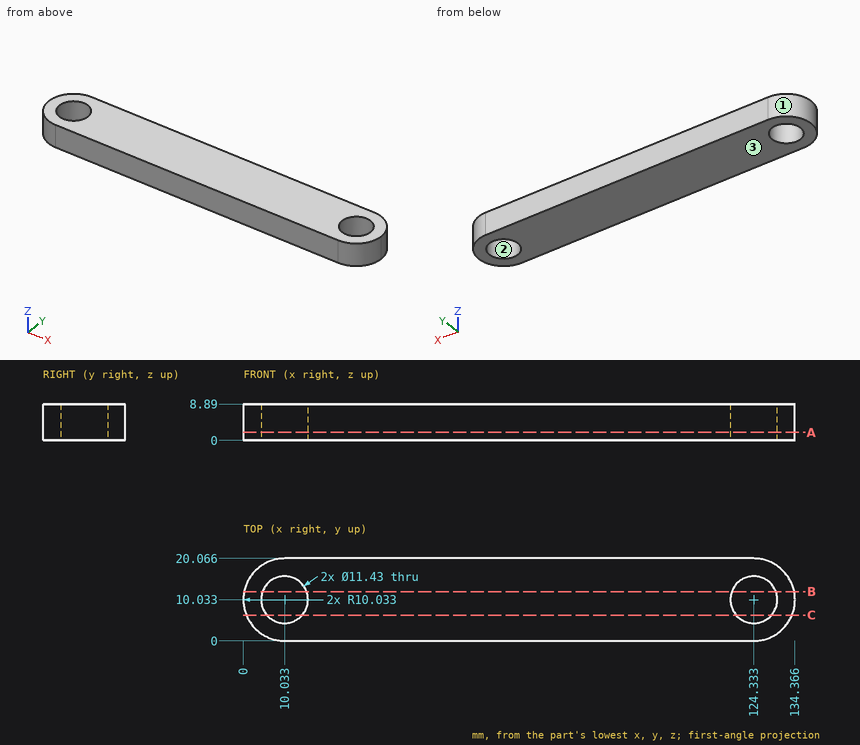
Input: dimensioned drawing with shaded views. Units: mm. Origin: part minimum x, y, z. Give positions to 0.01 mm unless a question says otherwise; leave off trailing zeros. Write each loop counter-clockwise with the first axis right and the second up, starting at its lowest first coordinate (ties: lowest second). Pieces come first, ordered by that corner, then holes. Notation, with made-up numbers: M -32.75,23.5 L 9.25,23.5 A24 cw 9.25,51.5 Z; hole C 60,-36 d3. An arc over 180 degrees is marked long. Write item = value, one per line. Start each with the question number.
1) Material intervals for line 1 along X through (y, z) = (5.5, 5.25); line 2 along X through (y, z) = (7, 7); line 3 along Y through (x, z) = (13, 2.5), sorted ascending. Write a range as [from, to].
2) Draft query along X for the marked faces 1, 2 and 3. Return one class per face: +X half, -X half, draft (parallel to the pull), parting line (faces both ways), or undercut.
3) Cut plane B-B on y = 12. Return the cut outline in (x, z).
4) Cut plane A-A on z = 2. Return the cut outline in (x, y) (3 decimals), then the cut area to 3 significant figures.
5) Cut plane C-C on y = 6.25. Return the cut outline in (x, z).
6) First-contact query: pin 1 Ø4 at (y, z) = (10.5, 5.5) entering from +X; pin 2 Ø3 at (y, z) = (13.5, 1) entering from +X; pin 3 Ø4 at (y, z) = (2, 4.5) entering from -X. Flat tips, straight axial feed; report the tip coordinate or a pass-through.
Solved:
q1.line_1 = [1.08, 6.55], [13.51, 120.85], [127.81, 133.28]
q1.line_2 = [0.47, 5.19], [14.88, 119.49], [129.18, 133.9]
q1.line_3 = [0, 5.15], [14.92, 20.07]
q2.face_1 = -X half
q2.face_2 = undercut
q2.face_3 = draft
q3.outline = M 0.19,0 L 4.67,0 L 4.67,8.89 L 0.19,8.89 Z; M 15.4,0 L 118.97,0 L 118.97,8.89 L 15.4,8.89 Z; M 129.7,0 L 134.17,0 L 134.17,8.89 L 129.7,8.89 Z
q4.outline = M 10.033,0 L 124.333,0 A10.033 ccw 124.333,20.066 L 10.033,20.066 A10.033 ccw Z; hole C 10.033,10.033 d11.43; hole C 124.333,10.033 d11.43
q4.area = 2,400 mm2
q5.outline = M 0.74,0 L 5.75,0 L 5.75,8.89 L 0.74,8.89 Z; M 14.32,0 L 120.05,0 L 120.05,8.89 L 14.32,8.89 Z; M 128.62,0 L 133.63,0 L 133.63,8.89 L 128.62,8.89 Z
q6.pin_1 = 134.37
q6.pin_2 = 134.17
q6.pin_3 = 2.02
